Design review of the part built by this model. Coordinates are the model's own, in mm. A direction names the side the tool comes from. Give positions to 0.01 mm unless a question says otherwise; leave off trailing zeros. Loops run counter-clockwise (first coordinate to the right, second up) from the corner with the lowest first, then second, coordinate; pieces in that order, holes last. Notation, with made-up numbers: (-14, 88) -> (15, 88) arc R36 cw to (15, 122) -> close; hole circle Ø1 at (24, 36.5). An arc over 180 degrees is marked (long way). Use a Markdown table: item, result. Add a question column.
1. Add section D-D (z = -3.25). State the section outline as (x, y) points.
2. Add section C-C (y = 2.6). State the section outline as (x, z) points, and give its area (3 significant figures).
3. To check wall thickness, follow line 1 (Y direction, x = 0, z = 2.75); line 2 (Y direction, x = 0, z = 0.5); line 3 (X direction, y = 2.6, z = -2). State the ranges of each line that lie inside material, in increasing order.
4. Add section B-B (z = 0). State the section outline as (x, y) points, and give its area (3 significant figures).
5. Draft analysis for pull direction X (two halves, no side actions). For faces 3 (the flat face through (0, 0.6, 0)), 4 (the cylindrical face through (0.1, 5.3, 0.1)), 5 (the flat face through (-0.2, 0.3, 6)), state which applies: pulls with the +X half, pulls with the -X half, needs draft (parallel to the pull), parting line crosses it, or undercut.
6. Add section A-A (x = 0). State the section outline as (y, z) points, and give its area (3 significant figures).
7. For pin 1 Ø1 at (y, z) = (2, 4) entering from -X; pin 2 Ø2 at (y, z) = (0.5, -4.5) entering from +X, all flat-tipped, find the tip position at first contact; note any pin that passes through.
8. For faces 1 (the flat face through (0, -3, 0)), 2 (the cylindrical face through (0.224, -1.479, 1.705)), list the 3-axis set-ups (+Z, -Z, +X, -X, +Y, -Y) from which the entire face can be reached by the end or side of a thin tool; tool diameter is ignored.
Autodesk Inventor part; units mm, degrees
ref_plane "YZ Plane" through (0, 0, 0) normal (1, 0, 0) x (0, 1, 0)
ref_plane "XZ Plane" through (0, 0, 0) normal (0, 1, 0) x (-1, 0, 0)
ref_plane "XY Plane" through (0, 0, 0) normal (0, 0, 1) x (1, 0, 0)
sketch "Szkic1" plane through (0, 0, 0) normal (0, 1, 0) x (-1, 0, 0)
  circle A0 centre (0, 0) radius 1.72
  line L0 (-2.5, 6) -> (2.5, 6)
  line L1 (2.5, 6) -> (2.5, -6)
  line L2 (2.5, -6) -> (-2.5, -6)
  line L3 (-2.5, -6) -> (-2.5, 6)
  line L4 (-2.5, 6) -> (2.5, -6) construction
  line L5 (2.5, 6) -> (-2.5, -6) construction
  dimension "d0" = 3.44
  dimension "d1" = 5
  dimension "d2" = 12
extrude "Wyciągnięcie proste1" add sketch "Szkic1" against normal blind 3 contours A0
extrude "Wyciągnięcie proste2" add sketch "Szkic1" along normal blind 0.6 contours A0 | L0 L1 L2 L3
sketch "Szkic2" plane through (-2.5, 0, 6) normal (0, 0, 1) x (1, 0, 0)
  line L0 (5, 0.6) -> (0, 0.6)
  line L1 (2.5, 0.6) -> (2.5, 2.6)
  line L2 (2.5, 0.6) -> (4.5, 0.6) construction
  circle A0 centre (2.5, 2.6) radius 2.2
  line L3 (0, 0.6) -> (5, 0.6)
  circle A1 centre (2.5, 2.6) radius 2.7
  point P0 (2.5, 0)
  point P1 (4.3138, 0.6)
  point P2 (0.6862, 0.6)
  point P3 (1.5835, 0.6)
  point P4 (3.4165, 0.6)
  dimension "d7" = 2
  dimension "d8" = 90
  dimension "d9" = 4.4
  dimension "d10" = 5.4
extrude "Wyciągnięcie proste3" add sketch "Szkic2" against normal up to surface (12 mm away) contours L0 A0 A1 picked at (4.985, 2.9942)
fillet "Zaokrąglenie1" radius 1 4 edges at (1.8138, 0.6, 0) (-1.8138, 0.6, 0) (2.5, 0.6, 0) (-2.5, 0.6, 0)
properties part number "wire_loop"
Taken from the geometry:
| question | item | result |
|---|---|---|
| 1 | outline | (-2.5, 0) -> (2.5, 0) -> (2.5, 0.39) arc R1 ccw to (2.44, 0.74) arc R1 cw to (2.46, 1.49) arc R2.7 ccw (long way) to (-2.46, 1.49) arc R1 cw to (-2.44, 0.74) arc R1 ccw to (-2.5, 0.39) -> close; hole (-0.92, 0.6) -> (0.92, 0.6) arc R2.2 ccw (long way) to start |
| 2 | outline | (-2.7, -6) -> (-2.2, -6) -> (-2.2, 6) -> (-2.7, 6) -> close; (2.2, -6) -> (2.7, -6) -> (2.7, 6) -> (2.2, 6) -> close |
| 2 | area | 12.0 mm^2 |
| 3 | line 1 | y = 0 to 0.6, 4.8 to 5.3 |
| 3 | line 2 | y = -3 to 0.6, 4.8 to 5.3 |
| 3 | line 3 | x = -2.7 to -2.2, 2.2 to 2.7 |
| 4 | outline | (-2.5, 0) -> (-1.72, 0) -> (-1.72, -3) -> (1.72, -3) -> (1.72, 0) -> (2.5, 0) -> (2.5, 0.39) arc R1 ccw to (2.44, 0.74) arc R1 cw to (2.46, 1.49) arc R2.7 ccw (long way) to (-2.46, 1.49) arc R1 cw to (-2.44, 0.74) arc R1 ccw to (-2.5, 0.39) -> close; hole (-0.92, 0.6) -> (0.92, 0.6) arc R2.2 ccw (long way) to start |
| 4 | area | 19.9 mm^2 |
| 5 | face 3 | undercut |
| 5 | face 4 | parting line crosses it |
| 5 | face 5 | needs draft |
| 6 | outline | (-3, -1.72) -> (0, -1.72) -> (0, -6) -> (0.6, -6) -> (0.6, 6) -> (0, 6) -> (0, 1.72) -> (-3, 1.72) -> close; (4.8, -6) -> (5.3, -6) -> (5.3, 6) -> (4.8, 6) -> close |
| 6 | area | 23.5 mm^2 |
| 7 | pin 1 | stops at x = -2.7 |
| 7 | pin 2 | stops at x = 2.5 |
| 8 | face 1 | +Z, -Z, +X, -X, -Y |
| 8 | face 2 | -Y |
